from build123d import *

# Parameters (mm, degrees)
EXTRUDE_1_DEPTH     = 2189
SKETCH_2_R          = 15.5
CUT_EXTRUDE_3_DEPTH = 2191.48419305
EXTRUDE_4_DEPTH     = 8
SKETCH_2_6_R        = 15.5
CUT_EXTRUDE_5_DEPTH = 2191.48419305
SKETCH_2_7_W        = 280
SKETCH_2_7_H        = 8
EXTRUDE_6_DEPTH     = 190


with BuildPart() as part:
    # Sketch 1 → Extrude 1 (new body)
    with BuildSketch(Plane.XY):
        Polygon((-150, 70), (-190, 70), (-190, -70), (-150, -70), (-150, -62), (-182, -62), (-182, 62), (-150, 62), align=None)
    extrude(amount=EXTRUDE_1_DEPTH)

    # Sketch 2 → Cut-Extrude 3 (cut, through all)
    with BuildSketch(Plane.ZY.offset(190)):
        with Locations(Location((50, 0, 0), (0, 0, 270))):
            Circle(SKETCH_2_R)
        with Locations(Location((170, 0, 0), (0, 0, 270))):
            Circle(SKETCH_2_R)
        with Locations(Location((2019, 0, 0), (0, 0, 90))):
            Circle(SKETCH_2_R)
        with Locations(Location((2139, 0, 0), (0, 0, 90))):
            Circle(SKETCH_2_R)
        Polygon((50, 70), (0, 20), (0, 70), align=None)
        Polygon((50, -70), (0, -20), (0, -70), align=None)
        Polygon((2189, -70), (2139, -70), (2189, -20), align=None)
        Polygon((2189, 70), (2139, 70), (2189, 20), align=None)
    extrude(amount=-CUT_EXTRUDE_3_DEPTH, mode=Mode.SUBTRACT)

    # Sketch 3 → Extrude 4 (add)
    with BuildSketch(Plane(origin=(-182, 0, 0), x_dir=(0, 0, -1), z_dir=(1, 0, 0))):
        Polygon((-2184, -17.928932188), (-2184, 17.928932188), (-2139.928932188, 62), (-1889, 62), (-1889, -62), (-2139.928932188, -62), align=None)
        Polygon((-5, -17.928932188), (-49.071067812, -62), (-300, -62), (-300, 62), (-49.071067812, 62), (-5, 17.928932188), align=None)
    extrude(amount=EXTRUDE_4_DEPTH)

    # Sketch 2_6 → Cut-Extrude 5 (cut, through all)
    with BuildSketch(Plane.ZY.offset(190)):
        with Locations(Location((50, 0, 0), (0, 0, 270))):
            Circle(SKETCH_2_6_R)
        with Locations(Location((170, 0, 0), (0, 0, 270))):
            Circle(SKETCH_2_6_R)
        with Locations(Location((2019, 0, 0), (0, 0, 180))):
            Circle(SKETCH_2_6_R)
        with Locations(Location((2139, 0, 0), (0, 0, 180))):
            Circle(SKETCH_2_6_R)
    extrude(amount=-CUT_EXTRUDE_5_DEPTH, mode=Mode.SUBTRACT)

    # Sketch 2_7 → Extrude 6 (add)
    with BuildSketch(Plane.ZY.offset(190)):
        with Locations((1094.5, 0)):
            Rectangle(SKETCH_2_7_W, SKETCH_2_7_H)
        with Locations((360, 0)):
            Rectangle(SKETCH_2_7_W, SKETCH_2_7_H)
        with Locations((1829, 0)):
            Rectangle(SKETCH_2_7_W, SKETCH_2_7_H)
    extrude(amount=-EXTRUDE_6_DEPTH)

    # Mirror 1: part across plane


with BuildPart() as part_1:
    add(part.part)
    add(part.part.mirror(Plane(origin=(0, -4, 1689), x_dir=(0, 0, 1), z_dir=(-1, 0, 0))))


solid = part_1.part
For this review, take the finished solid that the model builds, in its own axes (mm). A direction names the side the tool comes from. Round coordinates to 2 decimals unless told otherwise and drop trailing zeros. Write each loop counter-clockwise with the first axis right and the second up, starting at its lowest first coordinate (ties: lowest second). Pieces come first, ordered by that corner, then holes. Notation, with made-up numbers: (-2, 60) - (35, 60) arc R26 ccw to (35, 85) - close; hole circle Ø9 at (-24.5, 68). An arc over 180 degrees is marked (long way). Write item = value, one per line. Start each with the question number.
1. For faces 5 (the face through (170, -70, 1080)), 6 (the face through (182, -5, 4)), list the 3-axis set-ups (+Z, -Z, +X, -X, +Y, -Y) from which the entire face can be reached by the end or side of a thin tool; tool diameter is ignored.
2. Consider section A-A on z = 676.5. State the section outline as (x, y) points.
3. Wall thickness on L1, parallel to Z at x = -56.5, y = 0.5; L2, parallel to Z at x = 185, y = 0; L3, parallel to X at y = 59, z = 478.5: over which ranges is each line inside the solid? List them lowest first.
4. For pin 1 Ø6.5 at (x, y) = (177.5, 32.5) entering from -Z; pin 2 Ø25 at (y, z) = (0, 2019) entering from +X; pin 3 Ø6.5 at (x, y) = (-179, -5) entering from +Z; pin 4 Ø9 at (x, y) = (-176.5, 22) entering from +Z, all flat-tipped, find the tip position at first contact; note any pin that passes through.
5. Consider section B-B on x = 48. State the section outline as (y, z) points, plus the area to 3 significant figures.
6. Draft analysis for pull direction Y (two halves, no side actions). For faces 1 (the face through (-190, 1, 1079)), 2 (the face through (174, 1, 150)), 3 (the face through (184, 56, 2153)), 4 (the face through (-174, 15, 2034)), state which applies: released by +Y, released by -Y, zero draft, split by the parting line, or undercut.
7. Consider section C-C on y = -44. State the section outline as (x, z) points, plus the area to 3 significant figures.
Evaluation:
q1.face_5 = +Z, -Z, +X, -X, -Y
q1.face_6 = -Z
q2.outline = (-190, -70) - (-150, -70) - (-150, -62) - (-182, -62) - (-182, 62) - (-150, 62) - (-150, 70) - (-190, 70) - close; (150, -70) - (190, -70) - (190, 70) - (150, 70) - (150, 62) - (182, 62) - (182, -62) - (150, -62) - close
q3.L1 = 220 to 500, 954.5 to 1234.5, 1689 to 1969
q3.L2 = 0 to 34.5, 65.5 to 154.5, 185.5 to 2003.5, 2034.5 to 2123.5, 2154.5 to 2189
q3.L3 = -190 to -182, 182 to 190
q4.pin_1 = 16.32
q4.pin_2 = through
q4.pin_3 = 2189
q4.pin_4 = 2184
q5.outline = (-4, 220) - (4, 220) - (4, 500) - (-4, 500) - close; (-4, 954.5) - (4, 954.5) - (4, 1234.5) - (-4, 1234.5) - close; (-4, 1689) - (4, 1689) - (4, 1969) - (-4, 1969) - close
q5.area = 6,720 mm2
q6.face_1 = zero draft
q6.face_2 = undercut
q6.face_3 = released by +Y
q6.face_4 = undercut
q7.outline = (-190, 24) - (-182, 24) - (-182, 31.07) - (-174, 31.07) - (-174, 300) - (-182, 300) - (-182, 1889) - (-174, 1889) - (-174, 2157.93) - (-182, 2157.93) - (-182, 2165) - (-190, 2165) - close; (174, 31.07) - (182, 31.07) - (182, 24) - (190, 24) - (190, 2165) - (182, 2165) - (182, 2157.93) - (174, 2157.93) - (174, 1889) - (182, 1889) - (182, 300) - (174, 300) - close
q7.area = 42,900 mm2
